```python
from build123d import *

# Parameters (mm, degrees)
SKETCH1_W               = 31.75
SKETCH1_H               = 17.78
BOSS_EXTRUDE1_DEPTH     = 17.78
SKETCH3_R               = 6.4389
CUT_EXTRUDE1_DEPTH      = 13.97
CUT_EXTRUDE2_REACH      = 31.737
SKETCH2_R               = 3.6703
F_1_4_CLEARANCE_HOLE1_D = 6.5278


with BuildPart() as part:
    # Sketch1 → Boss-Extrude1 (new body)
    with BuildSketch(Plane(origin=(0, 0, 0), x_dir=(1, 0, 0), z_dir=(0, 1, 0))):
        Rectangle(SKETCH1_W, SKETCH1_H)
    extrude(amount=BOSS_EXTRUDE1_DEPTH)

    # Sketch3 → Cut-Extrude1 (cut)
    with BuildSketch(Plane(origin=(0, 0, -8.89), x_dir=(-1, 0, 0), z_dir=(0, 0, -1))):
        with Locations((6.35, 8.89)):
            Circle(SKETCH3_R)
    extrude(amount=-CUT_EXTRUDE1_DEPTH, mode=Mode.SUBTRACT)

    # Sketch2 → Cut-Extrude2 (cut, up to next)
    with BuildSketch(Plane.XY.offset(8.89), mode=Mode.PRIVATE) as cut_extrude2_sk1:
        with Locations((-6.35, 8.89)):
            Circle(SKETCH2_R)
    cut_extrude2_tool1 = extrude(cut_extrude2_sk1.sketch, amount=-CUT_EXTRUDE2_REACH, mode=Mode.PRIVATE) & part.part
    add(cut_extrude2_tool1.solids().sort_by_distance((-6.35, 8.89, 8.89))[0], mode=Mode.SUBTRACT)

    # 1/4 Clearance Hole1 (through all)
    with Locations(Plane(origin=(0, 17.78, 0), x_dir=(1, 0, 0), z_dir=(0, 1, 0))):
        with Locations((6.35, 0)):
            Hole(F_1_4_CLEARANCE_HOLE1_D / 2)


solid = part.part
```
Design review of the part built by this model. Coordinates are the model's own, in mm. A direction names the side the tool comes from. Coordinates: 2 decimals unless noted, no trailing zeros. Write each loop counter-clockwise with the first axis right and the second up, starting at its lowest first coordinate (ties: lowest second). Pieces come first, ordered by that corner, then holes.
1) Add section B-B (x = 6.35). Write out the cut boundary in (y, z).
2) Machinability: for faces 5 (the flat face through (0, 9, 8.89)), 6 (the flat face through (-9, 6, 5.08)), which of the approach directions +Z, -Z, +X, -X, +Y, -Y give a long, thin tool a straight path to every point of the face, cutting with its end or side? Answer none if there is none.
3) Add section A-A (y = 8.89). Write out the cut boundary in (x, z) (3 decimals).
4) Add section C-C (z = 0). Write out the cut boundary in (x, y) (3 decimals), plus the area to 3 significant figures.
5) Mouldability with a two-part tool opening along Y and no side actions: class faces 1 (the flat face through (3, 9, -8.89)), 2 (the flat face through (0, 0, 0)), 3 (the cylindrical face through (-2.96, 7.48, 7.01)), 4 (the cylindrical face through (-9.321, 3.178, -2.003)) as +Y half, -Y half, draft (parallel to the pull), parting line (faces both ways), or undercut.
6) Insertion check: pin 1 (4 mm diameter, centred on x = -6.5, y = 9, fed in from -Z). The pin has a flat end and moves straight along its axis. Give the tip position at first contact, or say it passes through.
7) Add section D-D (x = -6.35). Write out the cut boundary in (y, z).
8) To check wall thickness, follow L1, parallel to Y at x = -6.35, z = -2; L2, parallel to X at y = 9.5, z = -3 (3 decimals); L3, parallel to Z at x = 6.35, y = 5. State the ranges of each line that lie inside material, in increasing order.
Check result:
1. outline: (0, -8.89) - (17.78, -8.89) - (17.78, -3.26) - (0, -3.26) - close; (0, 3.26) - (17.78, 3.26) - (17.78, 8.89) - (0, 8.89) - close
2. face 5: +Z, +X, -X, +Y, -Y
2. face 6: -Z
3. outline: (-15.875, -8.89) - (-12.789, -8.89) - (-12.789, 5.08) - (-10.02, 5.08) - (-10.02, 8.89) - (-15.875, 8.89) - close; (-2.68, 5.08) - (0.089, 5.08) - (0.089, -8.89) - (15.875, -8.89) - (15.875, 8.89) - (-2.68, 8.89) - close; hole circle Ø6.528 at (6.35, 0)
4. outline: (-15.875, 0) - (3.086, 0) - (3.086, 17.78) - (-15.875, 17.78) - close; (9.614, 0) - (15.875, 0) - (15.875, 17.78) - (9.614, 17.78) - close; hole circle Ø12.878 at (-6.35, 8.89)
4. area: 318 mm2
5. face 1: draft
5. face 2: -Y half
5. face 3: undercut
5. face 4: undercut
6. pin 1: passes through
7. outline: (0, -8.89) - (2.45, -8.89) - (2.45, 5.08) - (5.22, 5.08) - (5.22, 8.89) - (0, 8.89) - close; (12.56, 5.08) - (15.33, 5.08) - (15.33, -8.89) - (17.78, -8.89) - (17.78, 8.89) - (12.56, 8.89) - close
8. L1: y = 0 to 2.45, 15.33 to 17.78
8. L2: x = -15.875 to -12.76, 0.06 to 5.064, 7.636 to 15.875
8. L3: z = -8.89 to -3.26, 3.26 to 8.89
